from build123d import *

# Parameters (mm, degrees)
SKETCH1_R           = 2.5
BOSS_EXTRUDE1_DEPTH = 0.8
SCALE1_SCALE        = 0.317565217


with BuildPart() as part:
    # Sketch1 → Boss-Extrude1 (new body)
    with BuildSketch(Plane.XY):
        with BuildLine():
            Line((-35, 0), (-35, -35))
            ThreePointArc((-35, -35), (0, -70), (35, -35))
            Line((35, -35), (35, 0))
            ThreePointArc((35, 0), (0, 35), (-35, 0))
        make_face()
        with Locations((-30.5, 0)):
            Circle(SKETCH1_R, mode=Mode.SUBTRACT)
        with Locations((0, 30.5)):
            Circle(SKETCH1_R, mode=Mode.SUBTRACT)
        with Locations((30.5, 0)):
            Circle(SKETCH1_R, mode=Mode.SUBTRACT)
        with Locations((30.5, -35)):
            Circle(SKETCH1_R, mode=Mode.SUBTRACT)
        with Locations((0, -65.5)):
            Circle(SKETCH1_R, mode=Mode.SUBTRACT)
        with Locations((-30.5, -35)):
            Circle(SKETCH1_R, mode=Mode.SUBTRACT)
        with BuildLine():
            Line((-26, 0), (-26, -35))
            ThreePointArc((-26, -35), (0, -61), (26, -35))
            Line((26, -35), (26, 0))
            ThreePointArc((26, 0), (0, 26), (-26, 0))
        make_face(mode=Mode.SUBTRACT)
    extrude(amount=BOSS_EXTRUDE1_DEPTH)


with BuildPart() as part_1:
    # Scale1: scaled about (0, -17.5, 0.4)
    add(part.part.scale(SCALE1_SCALE).moved(Location((0, -11.942608696, 0.272973913))))


solid = part_1.part
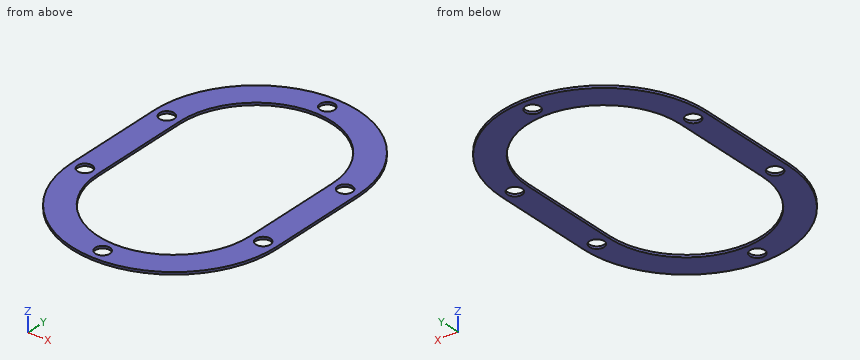
The model under review builds one solid part; all positions refer to its coordinate system, in mm. Round coordinates to 2 decimals unless told otherwise and drop trailing zeros. Write each loop counter-clockwise with the first axis right and the second up, starting at its lowest first coordinate (ties: lowest second). Pieces come first, ordered by that corner, then holes. Notation, with made-up numbers: M -9.5,9 L 1.5,9 A4 cw 1.5,14 Z; hole C -23.75,-16.5 d6. An arc over 180 degrees is marked long. Use a Markdown table: item, result. Add a question column.
Q1. We need section B-B, the plane y = -18. State the section outline as (x, z) points, plus the area to 3 significant figures.
Q2. Insertion check: pin 1 (5 mm diameter, centred on x = 3.5, y = -13.5, fed in from -Z). The pin has a flat end and moves straight along its axis. Give the tip position at first contact, or say it passes through.
Q3. To check wall thickness, follow line 1 (X direction, y = -12, z = 0.4); line 2 (Y direction, x = 0, z = 0.35); line 3 (X direction, y = -16, z = 0.35). State the ranges of each line that lie inside material, in increasing order.
Q4. We need section A-A, the plane x = 0. State the section outline as (y, z) points, plus the area to 3 significant figures.
Q5. We need section D-D, the plane z = 0.4. State the section outline as (x, y) points.
Q6. We need section C-C, the plane x = 5.5. State the section outline as (y, z) points, plus the area to 3 significant figures.
Findings below:
| question | item | result |
|---|---|---|
| 1 | outline | M -11.11,0.27 L -8.26,0.27 L -8.26,0.53 L -11.11,0.53 Z; M 8.26,0.27 L 11.11,0.27 L 11.11,0.53 L 8.26,0.53 Z |
| 1 | area | 1.45 mm² |
| 2 | pin 1 | passes through |
| 3 | line 1 | x = -11.11 to -10.48, -8.89 to -8.26, 8.26 to 8.89, 10.48 to 11.11 |
| 3 | line 2 | y = -34.17 to -33.54, -31.95 to -31.31, -3.69 to -3.05, -1.46 to -0.83 |
| 3 | line 3 | x = -11.11 to -8.26, 8.26 to 11.11 |
| 4 | outline | M -34.17,0.27 L -33.54,0.27 L -33.54,0.53 L -34.17,0.53 Z; M -31.95,0.27 L -31.31,0.27 L -31.31,0.53 L -31.95,0.53 Z; M -3.69,0.27 L -3.05,0.27 L -3.05,0.53 L -3.69,0.53 Z; M -1.46,0.27 L -0.83,0.27 L -0.83,0.53 L -1.46,0.53 Z |
| 4 | area | 0.645 mm² |
| 5 | outline | M -11.11,-23.06 A11.11 ccw 11.11,-23.06 L 11.11,-11.94 A11.11 ccw -11.11,-11.94 Z; hole C -9.69,-23.06 d1.59; hole C -9.69,-11.94 d1.59; hole M -8.26,-23.06 A8.26 ccw 8.26,-23.06 L 8.26,-11.94 A8.26 ccw -8.26,-11.94 Z; hole C 0,-32.74 d1.59; hole C 0,-2.26 d1.59; hole C 9.69,-23.06 d1.59; hole C 9.69,-11.94 d1.59 |
| 6 | outline | M -32.72,0.27 L -29.22,0.27 L -29.22,0.53 L -32.72,0.53 Z; M -5.78,0.27 L -2.28,0.27 L -2.28,0.53 L -5.78,0.53 Z |
| 6 | area | 1.78 mm² |
